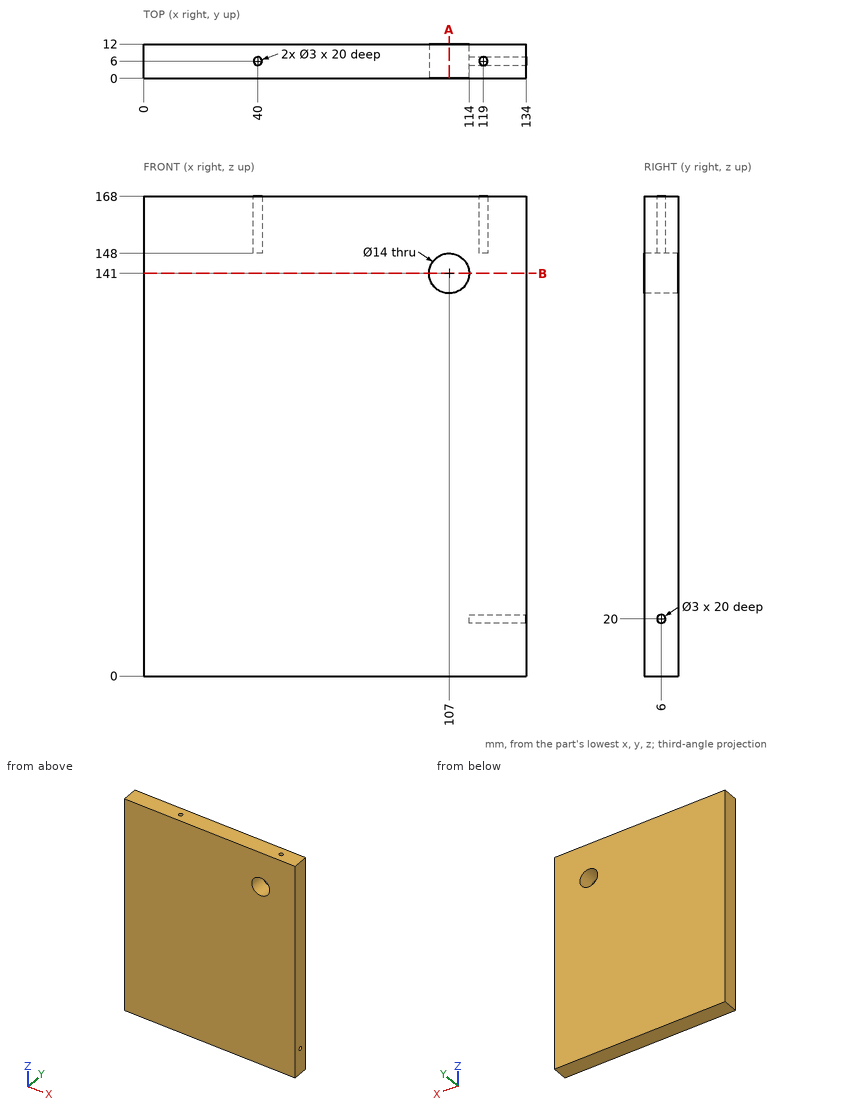
Geometry check sheet. Reference: drawing and pictorial views, mm from the part's lowest x, y, z. Round coordinates to 2 decimals unless told otherwise and drop trailing zeros. Order: outer loops, then holes, each group sorted by start corner. A loop starts at its lowest first (then second) coordinate and runs counter-clockwise, first axis right, second up. Notation, with made-up numbers: M 68,66 L 102,66 A14 ccw 102,80 Z; hole C -1.75,-8.75 d2. An arc over 180 degrees is marked long. Answer in a Markdown table with one row per item.
(1) Sectioned sample at B-B, the plane z = 141. Record the cut outline in (x, y).
Responses:
| item | result |
|---|---|
| outline | M 0,0 L 100,0 L 100,12 L 0,12 Z; M 114,0 L 134,0 L 134,12 L 114,12 Z |
(2) Sectioned sample at A-A, the plane x = 107. Record the cut outline in (y, z), and give its area (3 significant figures).
Responses:
| item | result |
|---|---|
| outline | M 0,0 L 12,0 L 12,134 L 0,134 Z; M 0,148 L 12,148 L 12,168 L 0,168 Z |
| area | 1,850 mm² |
(3) Scan lines: probe 1 along Z at (x, y) = (107, 6.5); probe 2 along X at (y, z) = (5.25, 152.5); probe 3 along Y at (x, z) = (40, 163.5). Record each from-to range of solid material in increasing order. Write a range as from..to.
Responses:
| item | result |
|---|---|
| probe 1 | z = 0..134, 148..168 |
| probe 2 | x = 0..38.7, 41.3..117.7, 120.3..134 |
| probe 3 | y = 0..4.5, 7.5..12 |
(4) Go/stop test with flat-tipped pins: P1, Ø0.9, axis at x = 119.5, y = 6.5, coming from the +Z side; P2, Ø2.5, axis at y = 6, z = 20, coming from the +X side. Record where each tip stops, or that it passes through.
Responses:
| item | result |
|---|---|
| P1 | stops at z = 148 |
| P2 | stops at x = 114 |
